Autodesk Inventor part; units mm, degrees
ref_plane "YZ Plane" through (0, 0, 0) normal (1, 0, 0) x (0, 1, 0)
ref_plane "XZ Plane" through (0, 0, 0) normal (0, 1, 0) x (-1, 0, 0)
ref_plane "XY Plane" through (0, 0, 0) normal (0, 0, 1) x (1, 0, 0)
sketch "スケッチ1" plane through (0, 0, 0) normal (1, 0, 0) x (0, 1, 0)
  line L0 (-110, 0) -> (-125, 0)
  line L1 (-110, 75) -> (-120, 75)
  arc A0 (-120, 75) -> (-120, -75) centre (2.1096, 0) ccw
  line L2 (0, 75) -> (0, -75)
  line L3 (-110, -75) -> (-120, -75)
  arc A1 (-110, 75) -> (-110, -75) centre (10, 0) ccw
  point P0 (0, 0)
  point P1 (0, 0)
  dimension "d0" = 150
  dimension "d2" = 0
  dimension "d4" = 10
  dimension "d35" = 20
revolve "回転1" add sketch "スケッチ1" angle 30 about axis through (0, 0, 75) along (0, 0, -1)
sketch "スケッチ2" plane through (0, -120, -75) normal (1, 0, 0) x (0, 0, -1)
  line L0 (-75, 120) -> (-97.7479, -9.0098) construction
  line L1 (-84.8481, 121.7365) -> (-107.596, -7.2733)
  line L2 (-87.8998, -10.7463) -> (-65.1519, 118.2635)
  arc A0 (-65.1519, 118.2635) -> (-84.8481, 121.7365) centre (-75, 120) ccw
  arc A1 (-107.596, -7.2733) -> (-87.8998, -10.7463) centre (-97.7479, -9.0098) ccw
  line L3 (-75, 120) -> (56, 120) construction
  point P0 (-86.374, 55.4951)
  dimension "d6" = 131
  dimension "d7" = 100
  dimension "d8" = 20
extrude "押し出し1" add sketch "スケッチ2" against normal blind 10
sketch "スケッチ3" plane through (0, -120, 75) normal (1, 0, 0) x (0, 0, -1)
  point P0 (75, 120)
  point P1 (75, 120)
hole "穴1" at (0, 0, 0) direction (-1, 0, 0) diameter 10 end through all
sketch "スケッチ5" plane through (1.0548, 1.8269, 0) normal (-0.8660254, 0.5, 0) x (-0.5, -0.8660254, 0)
  ellipse E0 centre (7.1096, 0) end of major axis (7.1096, -5) minor radius 4.3301
  line L0 (7.1096, 0) -> (186.6716, 22.6929)
  arc A0 (122.1096, -75) -> (122.1096, 75) centre (0, 0) ccw
  point P0 (2.1096, 0)
  point P1 (138, 16.5418)
  dimension "d27" = 138
hole "穴3" at (-67.9452, -117.6846, 16.5418) direction (0.8660254, -0.5, 0) diameter 4.8 depth 10
sketch "スケッチ6" plane through (0, 0, 0) normal (0, 1, 0) x (-1, 0, 0)
  line L0 (0, -75) -> (0, 12.9316)
  line L1 (0, -75) -> (55, -75)
  point P0 (0, 0)
  point P1 (5, -70)
  dimension "d36" = 5
  dimension "d37" = 5
hole "穴4" at (-5, 0, -70) direction (0, -1, 0) diameter 4.8 end through all
properties part number "受動歩行_ver4"
CAD build for the part. Positions are in the model's coordinates, mm. A direction names the side the tool comes from. Round coordinates to 2 decimals unless told otherwise and drop trailing zeros. Order: outer loops, then holes, each group sorted by start corner. A loop starts at its lowest first (then second) coordinate and runs counter-clockwise, first axis right, second up. Notation, with made-up numbers: (-12.75, 29) -> (19.25, 29) arc R13 cw to (19.25, 39) -> close; hole circle Ø8 at (11, 14). An arc over 180 degrees is marked (long way). Write item = value, one per line. Start each with the question number.
(1) Cut at A-A, the plane z = 0. State how many separate pieces and enclosed holes the cut face has, then the cut area to 3 significant figures.
(2) Which spindle directions (+Z, -Z, +X, -X, +Y, -Y) get a long thin tool onto all of the face, cutting with end or side? Do faces 1 (the flat face through (-30, -110, 75)), 2 (the flat face through (-59.3, -122.71, 16.51)). Say none if no direction does.
(3) Cut at B-B, the plane y = -76. List the corners of the cut face in (x, z).
(4) Probe line 1 (Z direction, x = -7, y = 0); line 2 (Z direction, x = -5, y = -120); line 3 (X direction, y = -114, z = -70). List the from-to ranges inside material, lowest first. Write a range as [from, to].
(5) Pin check, flat tips, straight feed: P1, Ø5, axis at x = -32.5, z = -12, coming from the +Y side; P2, Ø6, axis at x = -48.5, z = -19.5, coming from the +Y side; P3, Ø8, axis at y = -106.5, z = -47, coming from the -X side. Stop position of each tip, or through.
(6) Pull direction Z, two halves, no side cores. Call faces 3 (the cylindrical face through (-4.081, -117.899, -67.783)), 4 (the flat face through (-30, -110, -75)), 5 (the cylindrical face through (-4.9, 9.8, -2)): released by +Z, released by -Z, zero draft, split by the parting line, or undercut.
Model answer:
q1.separate_pieces = 3
q1.enclosed_holes = 0
q1.area = 1,270 mm2
q2.face_1 = +Z, +X, -X, +Y, -Y
q2.face_2 = none
q3.outline = (-10, 3.25) -> (0, 3.25) -> (0, 23.56) -> (-10, 23.56) -> close
q4.line_1 = [-10, -5], [5, 10.15]
q4.line_2 = [-74.83, -72.4], [-67.6, -55.66], [11, 31.31], [55.66, 74.83]
q4.line_3 = [-46.01, -7.4], [-2.6, 0]
q5.P1 = -126.2
q5.P2 = -119.46
q5.P3 = -63.8
q6.face_3 = undercut
q6.face_4 = released by -Z
q6.face_5 = split by the parting line
